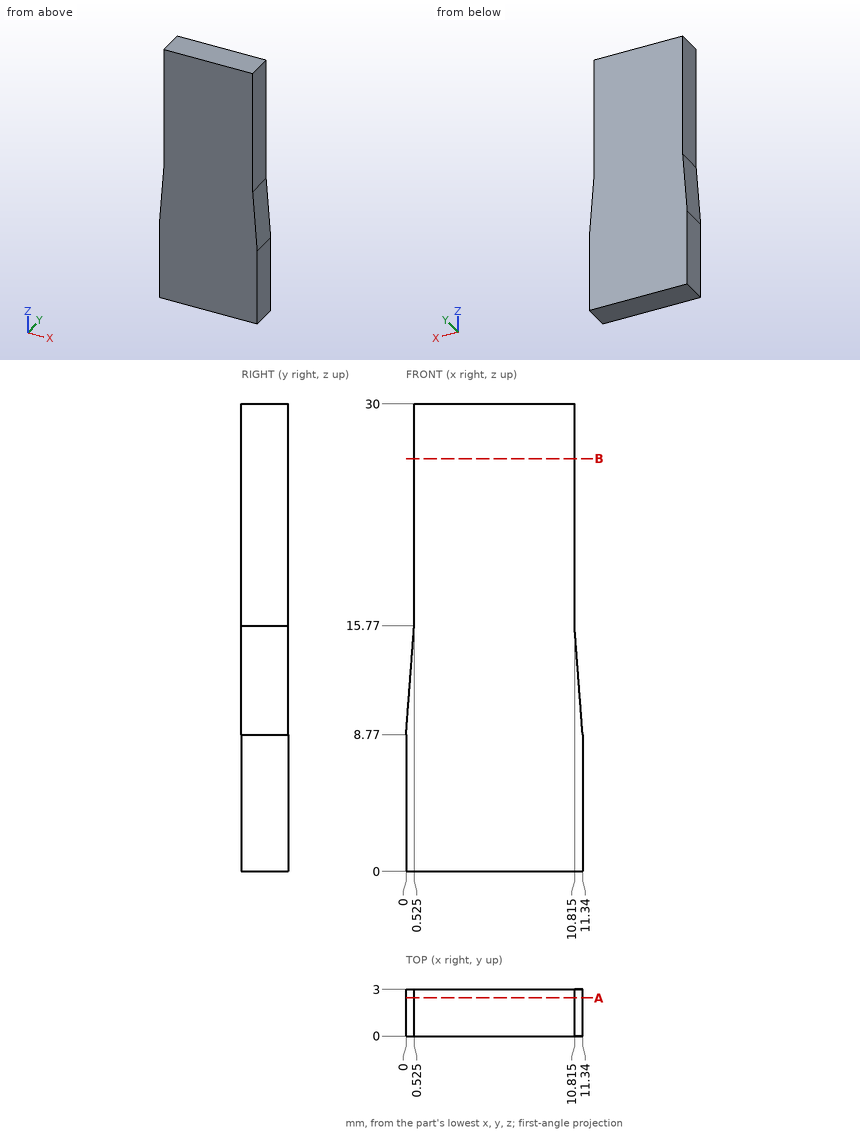
Design review of the part shown in the three views and the two pictorial views. Dimensions are in mm from the part's minimum x, y and z. Round coordinates to 2 decimals unless told otherwise and drop trailing zeros. Loops run counter-clockwise (first coordinate to the right, second up) from the corner with the lowest first, then second, coordinate; pieces in that order, holes last. Notation, with made-up numbers: (-28, 71) -> (-20, 71) arc R17 cw to (-20, 80) -> close; hole circle Ø7 at (7.5, 0). An arc over 180 degrees is marked (long way). Answer as a JSON object with one key per item and string values. Group by question number.
1) We need section B-B on z = 26.5. Write out the cut boundary in (x, y) (3 decimals), then the cut area to 3 significant figures.
2) For line 1 (X direction, y = 1.2, z = 23.75) (3 decimals); line 2 (X direction, y = 0.35, z = 13.75), list the stretches that pass through material, from the lowest coordinate up. Write a range as [from, to].
3) We need section A-A on y = 2.45. Write out the cut boundary in (x, z) (3 decimals), then the cut area to 3 significant figures.
4) For pin 1 Ø0.9 at (y, z) = (1, 24.5) entering from -X (3 decimals), flat-tipped, find the tip position at first contact; note if it passes through.
Result set:
{
 "1": {"outline": "(0.525, 0) -> (10.815, 0) -> (10.815, 3) -> (0.525, 3) -> close", "area": "30.9 mm²"},
 "2": {"line 1": "[0.525, 10.815]", "line 2": "[0.37, 10.97]"},
 "3": {"outline": "(0, 0) -> (11.34, 0) -> (11.34, 8.77) -> (10.815, 15.77) -> (10.815, 30) -> (0.525, 30) -> (0.525, 15.77) -> (0, 8.77) -> close", "area": "322 mm²"},
 "4": {"pin 1": "x = 0.525"}
}
